Could you check a few things on this model? Use its own coordinates, in mm. Round coordinates to 2 decimals unless told otherwise and drop trailing zeros. Order: outer loops, then holes, each group sorted by start corner. A loop starts at its lowest first (then second) coordinate and runs counter-clockwise, first axis right, second up. Notation, with made-up numbers: (11.25, -30.5) - (47.25, -30.5) arc R29 cw to (47.25, 3.5) - close; hole circle Ø3 at (64, 25). An arc over 180 degrees is marked (long way). Use one line per item in the form item = value.
from build123d import *

# Parameters (mm, degrees)
F0_W         = 40.3080582619
F0_H         = 5.9715644456
F1_DEPTH     = 668
F3_DEPTH     = 100
F5_DEPTH     = 5
F6_T1_DEPTH  = 716.1336390313
F9_DEPTH     = 4.9
F10_W        = 56.2156327069
F10_H        = 6.6376542673
F11_DEPTH    = 668
F12_T1_DEPTH = 831.8697028016


# Not quite as in the source:
# - a fillet or chamfer that OpenCascade refuses, or shapes differently, is made with other operations: its cross-section is extruded or revolved along the edge and cut away or added


with BuildPart() as f1:
    # F0 (on Top) → F1 (new body)
    with BuildSketch(Plane.XY):
        Rectangle(F0_W, F0_H)
    extrude(amount=F1_DEPTH)

    # F2 (on Top) → F3 (join)
    with BuildSketch(Plane.XY):
        Polygon((6.5744029718, -8.407556447), (10.5938451005, -1.2962352533), (8.407556447, 6.5744029718), (1.2962352533, 10.5938451005), (-6.5744029718, 8.407556447), (-10.5938451005, 1.2962352533), (-8.407556447, -6.5744029718), (-1.2962352533, -10.5938451005), align=None)
    extrude(amount=-F3_DEPTH)

    # F4 (on Top) → F5 (join)
    with BuildSketch(Plane.XY):
        Polygon((31.1715127681, -0.1368859226), (15.7043030704, 26.9268789703), (-15.4672096977, 27.0637648929), (-31.1715127681, 0.1368859226), (-15.7043030704, -26.9268789703), (15.4672096977, -27.0637648929), align=None)
    extrude(amount=F5_DEPTH)

    # F6: fillet of radius 270.3919189858 on 1 edges, made by hand

    # F6_s2 → F6_t1 (cut)
    with BuildSketch(Plane.XZ.offset(-358.0668195157)):
        with BuildLine():
            ThreePointArc((-20.1540291309, 668), (9.881896476, 599.7882231999), (20.1540291309, 525.9675850829))
            Line((20.1540291309, 525.9675850829), (20.1540291309, 668))
            Line((20.1540291309, 668), (-20.1540291309, 668))
        make_face()
    extrude(amount=F6_T1_DEPTH, mode=Mode.SUBTRACT)

    # F8 (on face) → F9 (join)
    with BuildSketch(Plane(origin=(0, 0, -100), x_dir=(1, 0, 0), z_dir=(0, 0, -1))):
        Polygon((30.9805478901, -0.0372380018), (15.5133381924, 27.0265268911), (-15.6581745757, 27.1634128136), (-31.3624776462, 0.2365338433), (-15.8952679485, -26.8272310495), (15.2762448196, -26.9641169721), align=None)
    extrude(amount=F9_DEPTH)

    # F10 (on offset) → F11 (join)
    with BuildSketch(Plane.XY.offset(-99)):
        Rectangle(F10_W, F10_H)
    extrude(amount=-F11_DEPTH)

    # F12: fillet of radius 270.392 on 1 edges, made by hand

    # F12_s2 → F12_t1 (cut)
    with BuildSketch(Plane.XZ.offset(-415.9348514008)):
        with BuildLine():
            ThreePointArc((-28.1078163534, -601.9535902931), (-13.6683607529, -689.132307188), (28.1078163534, -767))
            Line((28.1078163534, -767), (-28.1078163534, -767))
            Line((-28.1078163534, -767), (-28.1078163534, -601.9535902931))
        make_face()
    extrude(amount=F12_T1_DEPTH, mode=Mode.SUBTRACT)


solid = f1.part
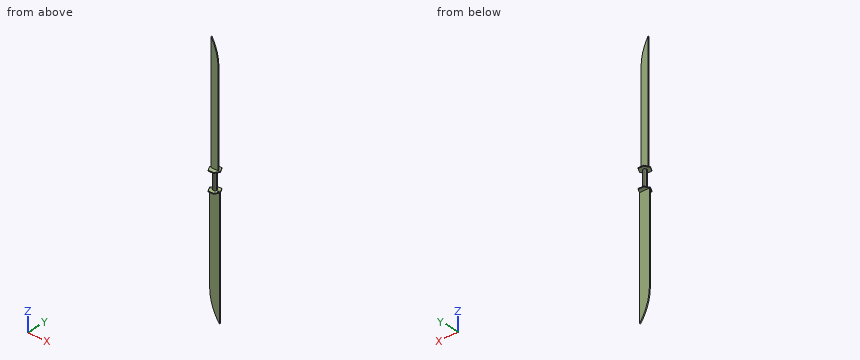
Item 1: Imagine slicing it at A-A on z = -300.5. Please give me the cut outline in (x, y).
Found:
outline = (-28.11, -3.32) - (28.11, -3.32) - (28.11, 3.32) - (-28.11, 3.32) - close
Item 2: I need wall thicknesses on L1, parallel to Z at x = 15, y = 19; L2, parallel to Y at x = 3.5, z = 279; L3, parallel to Y at x = 27.5, z = -566. Which ranges of each line are inside material? Lowest first, please.
Found:
L1 = -104.9 to -100, 0 to 5
L2 = -2.99 to 2.99
L3 = -3.32 to 3.32
Item 3: Imagine slicing it at B-B on z = -677. Please give me the cut outline in (x, y), plus the area to 3 significant figures.
Found:
outline = (-17.48, -3.32) - (28.11, -3.32) - (28.11, 3.32) - (-17.48, 3.32) - close
area = 303 mm2
Item 4: Will these pins go through, and if not, where does the flat tip stop? P1, Ø10, axis at y = -6, z = -158.5, coming from the -X side; P2, Ø0.5, axis at y = 0, z = -99.5, coming from the +X side; P3, Ø12, axis at x = -19, z = -461.5, coming from the -Y side; P4, Ø5, axis at y = 7, z = -267, coming from the +X side.
Found:
P1 = -28.11
P2 = 28.11
P3 = -3.32
P4 = through
